from build123d import *

# Parameters (mm, degrees)
SKETCH2_W                                           = 20
SKETCH2_H                                           = 30
BOSS_EXTRUDE1_DEPTH                                 = 30
SKETCH3_R                                           = 2.25
CUT_EXTRUDE2_DEPTH                                  = 19
SKETCH5_W                                           = 20
SKETCH5_H                                           = 30
BOSS_EXTRUDE2_DEPTH                                 = 5
SKETCH6_R                                           = 2.281198657
BOSS_EXTRUDE3_DEPTH                                 = 9
BOSS_EXTRUDE4_START                                 = 9
SKETCH7_R                                           = 2.25
BOSS_EXTRUDE4_DEPTH                                 = 9
BOSS_EXTRUDE6_DEPTH                                 = 9
SKETCH8_R                                           = 2.25
CUT_EXTRUDE3_DEPTH                                  = 40.37003937
CBORE_FOR_M4_HEX_SOCKET_HEAD_CAP_SCREW1_D           = 4.5
CBORE_FOR_M4_HEX_SOCKET_HEAD_CAP_SCREW1_DEPTH       = 35
CBORE_FOR_M4_HEX_SOCKET_HEAD_CAP_SCREW1_CBORE_D     = 8
CBORE_FOR_M4_HEX_SOCKET_HEAD_CAP_SCREW1_CBORE_DEPTH = 4
CUT_EXTRUDE6_DEPTH                                  = 10
CUT_EXTRUDE10_DEPTH                                 = 10
CUT_EXTRUDE11_DEPTH                                 = 10
SKETCH26_W                                          = 4
SKETCH26_H                                          = 10
CUT_EXTRUDE12_DEPTH                                 = 44.011626335
SKETCH32_W                                          = 30
SKETCH32_H                                          = 35
BOSS_EXTRUDE15_DEPTH                                = 3
SKETCH33_W                                          = 4
SKETCH33_H                                          = 10
BOSS_EXTRUDE16_DEPTH                                = 3
SKETCH34_W                                          = 3
SKETCH34_H                                          = 30
BOSS_EXTRUDE17_DEPTH                                = 20
SKETCH35_W                                          = 3
SKETCH35_H                                          = 30
BOSS_EXTRUDE18_DEPTH                                = 20
SKETCH37_R                                          = 1.75
CUT_EXTRUDE15_DEPTH                                 = 47.108567534
FILLET1_R_R                                         = 2
FILLET2_R_R                                         = 2


with BuildPart() as part:
    # Sketch2 → Boss-Extrude1 (new body)
    with BuildSketch(Plane(origin=(0, 0, 0), x_dir=(1, 0, 0), z_dir=(0, 1, 0))):
        Rectangle(SKETCH2_W, SKETCH2_H)
    extrude(amount=BOSS_EXTRUDE1_DEPTH)

    # Sketch3 → Cut-Extrude2 (cut)
    with BuildSketch(Plane(origin=(0, 30, 0), x_dir=(1, 0, 0), z_dir=(0, 1, 0))):
        with BuildLine():
            Line((-1.5, -15), (10, -15))
            Line((10, -15), (10, -1))
            Line((10, -1), (5.5, -1))
            ThreePointArc((5.5, -1), (3.403805654, -1.321229959), (1.5, -2.255437353))
            Line((1.5, -2.255437353), (1.5, 4))
            ThreePointArc((1.5, 4), (1.178770041, 6.096194346), (0.244562647, 8))
            Line((0.244562647, 8), (10, 8))
            Line((10, 8), (10, 11))
            Line((10, 11), (-10, 11))
            Line((-10, 11), (-10, -3))
            Line((-10, -3), (-5.5, -3))
            ThreePointArc((-5.5, -3), (-3.403805654, -2.678770041), (-1.5, -1.744562647))
            Line((-1.5, -1.744562647), (-1.5, -15))
        make_face()
        with Locations(Location((5.5, -8, 0), (0, 0, 270))):
            Circle(SKETCH3_R, mode=Mode.SUBTRACT)
        with Locations(Location((-5.5, 4, 0), (0, 0, 270))):
            Circle(SKETCH3_R, mode=Mode.SUBTRACT)
    extrude(amount=-CUT_EXTRUDE2_DEPTH, mode=Mode.SUBTRACT)

    # Sketch5 → Boss-Extrude2 (add)
    with BuildSketch(Plane(origin=(0, 30, 0), x_dir=(1, 0, 0), z_dir=(0, 1, 0))):
        Rectangle(SKETCH5_W, SKETCH5_H)
    extrude(amount=BOSS_EXTRUDE2_DEPTH)

    # Sketch6 → Boss-Extrude3 (add)
    with BuildSketch(Plane.XZ.offset(-30)):
        with BuildLine():
            Line((1.5, 2.255437353), (1.5, 15))
            Line((1.5, 15), (10, 15))
            Line((10, 15), (10, 1))
            Line((10, 1), (5.5, 1))
            ThreePointArc((5.5, 1), (3.403805654, 1.321229959), (1.5, 2.255437353))
        make_face()
        with Locations(Location((5.5, 8, 0), (0, 0, 270))):
            Circle(SKETCH6_R, mode=Mode.SUBTRACT)
    extrude(amount=BOSS_EXTRUDE3_DEPTH)

    # Sketch7 → Boss-Extrude4 (add)
    with BuildSketch(Plane(origin=(0, 11, 0), x_dir=(1, 0, 0), z_dir=(0, 1, 0)).offset(BOSS_EXTRUDE4_START)):
        with BuildLine():
            ThreePointArc((1.5, 4), (1.178770041, 6.096194346), (0.244562647, 8))
            Line((0.244562647, 8), (-10, 8))
            Line((-10, 8), (-10, -3))
            Line((-10, -3), (-5.5, -3))
            ThreePointArc((-5.5, -3), (-3.403805654, -2.678770041), (-1.5, -1.744562647))
            Line((-1.5, -1.744562647), (-1.5, -8))
            ThreePointArc((-1.5, -8), (-0.704836823, -4.759629651), (1.5, -2.255437353))
            Line((1.5, -2.255437353), (1.5, 4))
        make_face()
        with Locations((-5.5, 4)):
            Circle(SKETCH7_R, mode=Mode.SUBTRACT)
    extrude(amount=-BOSS_EXTRUDE4_DEPTH)

    # Sketch15 → Boss-Extrude6 (add)
    with BuildSketch(Plane.XZ.offset(-30)):
        with BuildLine():
            Line((10, -8), (10, -11))
            Line((10, -11), (-5.5, -11))
            ThreePointArc((-5.5, -11), (-2.259629651, -10.204836823), (0.244562647, -8))
            Line((0.244562647, -8), (10, -8))
        make_face()
    extrude(amount=BOSS_EXTRUDE6_DEPTH)

    # Sketch8 → Cut-Extrude3 (cut, through all)
    with BuildSketch(Plane(origin=(0, 35, 0), x_dir=(1, 0, 0), z_dir=(0, 1, 0))):
        with Locations(Location((5.5, -8, 0), (0, 0, 270))):
            Circle(SKETCH8_R)
        with Locations(Location((-5.5, 4, 0), (0, 0, 270))):
            Circle(SKETCH8_R)
    extrude(amount=-CUT_EXTRUDE3_DEPTH, mode=Mode.SUBTRACT)

    # CBORE for M4 Hex Socket Head Cap Screw1
    with Locations(Plane(origin=(0, 35, 0), x_dir=(1, 0, 0), z_dir=(0, 1, 0))):
        with Locations((5.5, -8), (-5.5, 4)):
            CounterBoreHole(CBORE_FOR_M4_HEX_SOCKET_HEAD_CAP_SCREW1_D / 2, CBORE_FOR_M4_HEX_SOCKET_HEAD_CAP_SCREW1_CBORE_D / 2, CBORE_FOR_M4_HEX_SOCKET_HEAD_CAP_SCREW1_CBORE_DEPTH, depth=CBORE_FOR_M4_HEX_SOCKET_HEAD_CAP_SCREW1_DEPTH)

    # Sketch14 → Cut-Extrude6 (cut)
    with BuildSketch(Plane.XZ):
        Polygon((5.5, 3.814210548), (9.125, 5.907105274), (9.125, 10.092894726), (5.5, 12.185789452), (1.875, 10.092894726), (1.875, 5.907105274), align=None)
        Polygon((-5.5, -8.185789452), (-1.875, -6.092894726), (-1.875, -1.907105274), (-5.5, 0.185789452), (-9.125, -1.907105274), (-9.125, -6.092894726), align=None)
    extrude(amount=-CUT_EXTRUDE6_DEPTH, mode=Mode.SUBTRACT)

    # Sketch24 → Cut-Extrude10 (cut)
    with BuildSketch(Plane(origin=(0, 11, 0), x_dir=(1, 0, 0), z_dir=(0, 1, 0))):
        with BuildLine():
            Line((-2.5, -16), (11, -16))
            Line((11, -16), (11, 0))
            Line((11, 0), (5.5, 0))
            ThreePointArc((5.5, 0), (-0.156854249, -2.343145751), (-2.5, -8))
            Line((-2.5, -8), (-2.5, -16))
        make_face()
    extrude(amount=CUT_EXTRUDE10_DEPTH, mode=Mode.SUBTRACT)

    # Sketch25 → Cut-Extrude11 (cut)
    with BuildSketch(Plane.XZ.offset(-30)):
        with BuildLine():
            Line((-10, -12), (-10, 4))
            Line((-10, 4), (-5.5, 4))
            ThreePointArc((-5.5, 4), (-3.9718619, 3.85269342), (-2.5, 3.416198487))
            Line((-2.5, 3.416198487), (-2.5, 15))
            Line((-2.5, 15), (2.5, 15))
            Line((2.5, 15), (2.5, -4))
            ThreePointArc((2.5, -4), (0.156854249, -9.656854249), (-5.5, -12))
            Line((-5.5, -12), (-10, -12))
        make_face()
    extrude(amount=CUT_EXTRUDE11_DEPTH, mode=Mode.SUBTRACT)

    # Sketch26 → Cut-Extrude12 (cut, through all)
    with BuildSketch(Plane.ZY.offset(10)):
        with Locations((-10, 16)):
            Rectangle(SKETCH26_W, SKETCH26_H)
    extrude(amount=-CUT_EXTRUDE12_DEPTH, mode=Mode.SUBTRACT)

    # Sketch32 → Boss-Extrude15 (add)
    with BuildSketch(Plane.ZY.offset(10)):
        with Locations((0, 17.5)):
            Rectangle(SKETCH32_W, SKETCH32_H)
        Polygon((-12, 11), (-8, 11), (-8, 20), (4, 20), (4, 30), (-12, 30), align=None, mode=Mode.SUBTRACT)
    extrude(amount=BOSS_EXTRUDE15_DEPTH)

    # Sketch33 → Boss-Extrude16 (add)
    with BuildSketch(Plane(origin=(10, 0, 0), x_dir=(0, 0, -1), z_dir=(1, 0, 0))):
        Polygon((15, 35), (15, 0), (-15, 0), (-15, 11), (0, 11), (0, 21), (-15, 21), (-15, 35), align=None)
        with Locations((10, 16)):
            Rectangle(SKETCH33_W, SKETCH33_H, mode=Mode.SUBTRACT)
    extrude(amount=BOSS_EXTRUDE16_DEPTH)

    # Sketch34 → Boss-Extrude17 (add)
    with BuildSketch(Plane.XZ):
        with Locations((-11.5, 0)):
            Rectangle(SKETCH34_W, SKETCH34_H)
    extrude(amount=BOSS_EXTRUDE17_DEPTH)

    # Sketch35 → Boss-Extrude18 (add)
    with BuildSketch(Plane.XZ):
        with Locations((11.5, 0)):
            Rectangle(SKETCH35_W, SKETCH35_H)
    extrude(amount=BOSS_EXTRUDE18_DEPTH)

    # Sketch37 → Cut-Extrude15 (cut, through all)
    with BuildSketch(Plane.ZY.offset(13)):
        with Locations((-10, -10)):
            Circle(SKETCH37_R)
        with Locations((10, -10)):
            Circle(SKETCH37_R)
    extrude(amount=-CUT_EXTRUDE15_DEPTH, mode=Mode.SUBTRACT)

    # Fillet1-r
    fillet1_r_edges = [part.edges().sort_by_distance(p)[0] for p in [
        (-13, 7.5, 15),
        (-13, 35, 0),
        (13, 35, 0),
        (13, 28, 15),
        (13, -4.5, 15),
        (-13, -20, 0),
        (-11.5, -20, 15),
        (13, -20, 0),
        (11.5, -20, 15),
        (0, 35, 15),
    ]]
    fillet(fillet1_r_edges, radius=FILLET1_R_R)

    # Fillet2-r
    fillet2_r_edges = [part.edges().sort_by_distance(p)[0] for p in [
        (-2.5, 20.5, 15),
        (2.5, 25.5, 15),
        (-2.5, 25, 3.416198487),
        (-13, 20.5, -12),
        (-13, 15.5, -8),
        (-13, 25, 4),
        (13, 16, 0),
        (13, 16, -8),
        (13, 16, -12),
    ]]
    fillet(fillet2_r_edges, radius=FILLET2_R_R)


solid = part.part
Can you work these out from the model? Positions are in its coordinate system, mm. A direction names the side the tool comes from. Round coordinates to 2 decimals unless told otherwise and drop trailing zeros. Write each loop counter-clockwise with the first axis right and the second up, starting at its lowest first coordinate (ties: lowest second). Pieces come first, ordered by that corner, then holes. Notation, with made-up numbers: M -5.75,81 L 39.25,81 A27 ccw 39.25,116 Z; hole C 27.5,62.25 d1. An arc over 180 degrees is marked long. Use a Markdown table: item, result.
Item 1: We'd pull the mould along X, two halves only. Please class faces 4 (the face through (-12.43, 20.37, -12.6)), 5 (the face through (6.1, 11, 10.4)), 6 (the face through (-9.125, 5, -4)), 7 (the face through (12.43, 16.07, -12.6)): released by +X, released by -X, zero draft, split by the parting line, or undercut.
Found:
| item | result |
|---|---|
| face 4 | released by -X |
| face 5 | zero draft |
| face 6 | undercut |
| face 7 | released by +X |
Item 2: For pin 1 Ø7.5 at (x, z) = (5.5, 8) entering from +Y; pin 2 Ø3.5 at (x, z) = (-5.5, -4) entering from +Y; pin 3 Ø3 at (x, z) = (6.5, -7) entering from -Y, each with a flat end and sliding along its axis, tell me the tip position at first contact or that it passes through.
Found:
| item | result |
|---|---|
| pin 1 | stops at y = 31 |
| pin 2 | passes through |
| pin 3 | stops at y = 0 |
Item 3: I want a section at A-A (y = -10). List the corners of the cut face in (x, z) for me.
Found:
| item | result |
|---|---|
| outline | M -13,-15 L -10,-15 L -10,-11.75 L -13,-11.75 Z; M -13,-8.25 L -10,-8.25 L -10,8.25 L -13,8.25 Z; M -13,11.75 L -10,11.75 L -10,15 L -11,15 A2 ccw -13,13 Z; M 10,-15 L 13,-15 L 13,-11.75 L 10,-11.75 Z; M 10,-8.25 L 13,-8.25 L 13,8.25 L 10,8.25 Z; M 10,11.75 L 13,11.75 L 13,13 A2 ccw 11,15 L 10,15 Z |
Item 4: I want a section at D-D (y = 7.5). List the corners of the cut face in (x, z) for me (3 decimals).
Found:
| item | result |
|---|---|
| outline | M -13,-15 L 13,-15 L 13,13 A2 ccw 11,15 L -11,15 A2 ccw -13,13 Z; hole M -9.125,-6.093 L -5.5,-8.186 L -1.875,-6.093 L -1.875,-1.907 L -5.5,0.186 L -9.125,-1.907 Z; hole M 1.875,5.907 L 5.5,3.814 L 9.125,5.907 L 9.125,10.093 L 5.5,12.186 L 1.875,10.093 Z |
Item 5: I want a section at C-C (z = -10). List the corners of the cut face in (x, y) for me.
Found:
| item | result |
|---|---|
| outline | M -13,-18 A2 ccw -11,-20 L -10,-20 L -10,-11.75 L -13,-11.75 Z; M -13,-8.25 L -10,-8.25 L -10,0 L 10,0 L 10,-8.25 L 13,-8.25 L 13,11 L -13,11 Z; M -13,30 L -0.21,30 L -0.21,21 L 13,21 L 13,33 A2 ccw 11,35 L -11,35 A2 ccw -13,33 Z; M 10,-20 L 11,-20 A2 ccw 13,-18 L 13,-11.75 L 10,-11.75 Z |
Item 6: If I drill on line 1 along X through (y, z) = (-1.5, 3.75); line 2 along X through (y, z) = (30.7, 8); line 3 along X through (y, z) = (29, 9.5), over which ranges is the centre line in solid material (lowest first)? Write a range as [from, to].
Found:
| item | result |
|---|---|
| line 1 | x = [-13, -10], [10, 13] |
| line 2 | x = [-13, 3.25], [7.75, 13] |
| line 3 | x = [-13, -2.5], [2.5, 3.78], [7.22, 13] |
Item 7: Which directions (+Z, -Z, +X, -X, +Y, -Y) give clear straight access to the entire face, cutting with the end or side of a thin tool? Please do faces 1 (the face through (7.338, 4.93, 11.125)), 2 (the face through (10, -10, 0)), 3 (the face through (2.5, 25, 5)).
Found:
| item | result |
|---|---|
| face 1 | -Y |
| face 2 | +Z, -Z, -Y |
| face 3 | +Z |
Item 8: I want a section at B-B (x = 6.25). State how many separate pieces and enclosed holes the cut face has, and give its area (3 significant figures).
Found:
| item | result |
|---|---|
| separate pieces | 3 |
| enclosed holes | 1 |
| area | 705 mm2 |
